from build123d import *

# Parameters (mm, degrees)
SKETCH_1_W          = 32
SKETCH_1_H          = 34
SKETCH_1_R          = 3.388194149
SKETCH_1_R_2        = 1.2
SKETCH_1_R_3        = 5.5
EXTRUDE_1_DEPTH     = 13.5
EXTRUDE_START       = 3
SKETCH_1_26_R       = 1.2
EXTRUDE_3_DEPTH     = 10.5
EXTRUDE_START_2     = -3
SKETCH_1_25_W       = 32
SKETCH_1_25_H       = 34
SKETCH_1_25_R       = 3.388194149
SKETCH_1_25_R_2     = 1.2
EXTRUDE_2_DEPTH     = 3
SKETCH_2_W          = 4
SKETCH_2_H          = 7
SKETCH_2_W_2        = 5
SKETCH_2_H_2        = 2
EXTRUDE_4_DEPTH     = 4
SKETCH_2_3_R        = 1.5
CUT_EXTRUDE_1_DEPTH = 35.091787867
CUT_EXTRUDE_START   = -16.5
SKETCH_2_4_R        = 2.25
CUT_EXTRUDE_2_DEPTH = 14.5
SKETCH_3_R          = 0.75
CUT_EXTRUDE_3_DEPTH = 4
SKETCH_1_27_R       = 3.388194149
EXTRUDE_5_DEPTH     = 16.5


with BuildPart() as part:
    # 草图1 → 凸台-拉伸1 (new body)
    with BuildSketch(Plane(origin=(0, 0, 0), x_dir=(1, 0, 0), z_dir=(0, 1, 0))):
        with Locations((3, 6)):
            Rectangle(SKETCH_1_W, SKETCH_1_H)
        with Locations(Location((11.473501894, 0, 0), (0, 0, 270))):
            Circle(SKETCH_1_R, mode=Mode.SUBTRACT)
        with Locations(Location((-3.489130435, 11.48154906, 0), (0, 0, 270))):
            Circle(SKETCH_1_R_2, mode=Mode.SUBTRACT)
        with Locations(Location((0, 0, 0), (0, 0, 270))):
            Circle(SKETCH_1_R_3, mode=Mode.SUBTRACT)
    extrude(amount=EXTRUDE_1_DEPTH)

    # 草图1<26> → 凸台-拉伸3 (add)
    with BuildSketch(Plane(origin=(0, 0, 0), x_dir=(1, 0, 0), z_dir=(0, 1, 0)).offset(EXTRUDE_START)):
        with Locations(Location((-3.489130435, 11.48154906, 0), (0, 0, 270))):
            Circle(SKETCH_1_26_R)
    extrude(amount=EXTRUDE_3_DEPTH)

    # 草图1<25> → 凸台-拉伸2 (add)
    with BuildSketch(Plane(origin=(0, 0, 0), x_dir=(1, 0, 0), z_dir=(0, 1, 0)).offset(EXTRUDE_START_2)):
        with Locations((3, 6)):
            Rectangle(SKETCH_1_25_W, SKETCH_1_25_H)
        with Locations(Location((11.473501894, 0, 0), (0, 0, 270))):
            Circle(SKETCH_1_25_R, mode=Mode.SUBTRACT)
        with BuildLine():
            ThreePointArc((5.276856444, 1.550737267), (6.181423335, 0.479588939), (5.452898061, -0.718263692))
            ThreePointArc((5.452898061, -0.718263692), (-1.935120147, -5.148330799), (-4.575965094, 3.051318314))
            ThreePointArc((-4.575965094, 3.051318314), (-5.960597826, 19.614312977), (2.104497703, 5.081445603))
            ThreePointArc((2.104497703, 5.081445603), (4.091157856, 3.67592538), (5.276856444, 1.550737267))
        make_face(mode=Mode.SUBTRACT)
        with Locations(Location((8.010869565, 11.48154906, 0), (0, 0, 270))):
            Circle(SKETCH_1_25_R_2, mode=Mode.SUBTRACT)
    extrude(amount=EXTRUDE_2_DEPTH)

    # 草图2 → 凸台-拉伸4 (add)
    with BuildSketch(Plane(origin=(0, 13.5, 0), x_dir=(1, 0, 0), z_dir=(0, 1, 0))):
        with Locations((-15, 9.3)):
            Rectangle(SKETCH_2_W, SKETCH_2_H)
        with Locations((0.1, -12)):
            Rectangle(SKETCH_2_W_2, SKETCH_2_H_2)
    extrude(amount=-EXTRUDE_4_DEPTH)

    # 草图2<3> → 切除-拉伸1 (cut, through all)
    with BuildSketch(Plane(origin=(0, 13.5, 0), x_dir=(1, 0, 0), z_dir=(0, 1, 0))):
        with Locations(Location((-13.25, 9.25, 0), (0, 0, 270))):
            Circle(SKETCH_2_3_R)
        with Locations(Location((0, -9.25, 0), (0, 0, 270))):
            Circle(SKETCH_2_3_R)
        with Locations(Location((13.25, 9.25, 0), (0, 0, 270))):
            Circle(SKETCH_2_3_R)
    extrude(amount=-CUT_EXTRUDE_1_DEPTH, mode=Mode.SUBTRACT)

    # 草图2<4> → 切除-拉伸2 (cut)
    with BuildSketch(Plane(origin=(0, 13.5, 0), x_dir=(1, 0, 0), z_dir=(0, 1, 0)).offset(CUT_EXTRUDE_START)):
        with Locations(Location((-13.25, 9.25, 0), (0, 0, 83.620629792))):
            Circle(SKETCH_2_4_R)
        with Locations(Location((13.25, 9.25, 0), (0, 0, 270))):
            Circle(SKETCH_2_4_R)
        with Locations(Location((0, -9.25, 0), (0, 0, 308.942441269))):
            Circle(SKETCH_2_4_R)
    extrude(amount=CUT_EXTRUDE_2_DEPTH, mode=Mode.SUBTRACT)

    # 草图3 → 切除-拉伸3 (cut)
    with BuildSketch(Plane.XZ.offset(3)):
        with Locations(Location((-10, 8, 0), (0, 0, 270))):
            Circle(SKETCH_3_R)
        with Locations(Location((17, -21, 0), (0, 0, 270))):
            Circle(SKETCH_3_R)
        with Locations(Location((16, 8, 0), (0, 0, 270))):
            Circle(SKETCH_3_R)
    extrude(amount=-CUT_EXTRUDE_3_DEPTH, mode=Mode.SUBTRACT)

    # 草图1<27> → 凸台-拉伸5 (add, through all)
    with BuildSketch(Plane(origin=(0, 0, 0), x_dir=(1, 0, 0), z_dir=(0, 1, 0)).offset(EXTRUDE_START_2)):
        with Locations((11.473501894, 0)):
            Circle(SKETCH_1_27_R)
    extrude(amount=EXTRUDE_5_DEPTH)


solid = part.part
Could you check a few things on this model? Use its own coordinates, in mm. A direction names the side the tool comes from. Coordinates: 2 decimals unless noted, no trailing zeros. Order: outer loops, then holes, each group sorted by start corner. A loop starts at its lowest first (then second) coordinate and runs counter-clockwise, first axis right, second up.
Q1. Which directions (+Z, -Z, +X, -X, +Y, -Y) give clear straight access to the entire face, cutting with the end or side of a thin tool? Please do faces 1 (the cylindrical face through (-13.18, 12.51, -10.75)), 2 (the flat face through (-2.4, 12, 12)), 3 (the cylindrical face through (9.2, -1.52, -11.64)), 4 (the flat face through (2.6, 12, 12)), 5 (the flat face through (-15, 12, -12.8)).
Q2. Thinking about a two-plate mould opening in Z: for faces 6 (the flat face through (0, 12, 13)), 7 (the flat face through (5, 13.5, -5)), 8 (the cylindrical face through (6.18, -1.52, -0.5)), which applies, released by +Z, released by -Z, zero draft, split by the parting line, or undercut?
Q3. Please list where these lines run through material, in increasing order: L1, parallel to Z at x = 0, y = 10; L2, parallel to X at y = 0.25, z = 8; L3, parallel to X at y = 2.5, z = 0.
Q4. Suppose I cut it at B-B on y = 5.75. Please give me the cut outline in (x, z).
Q5. Suppose I cut it at C-C on x = 13.25. Please give me the cut outline in (y, z).
Q6. Suppose I cut it at D-D on z = -9.25. Please give me the cut outline in (x, y).
Q7. Will these pins go through, and if not, where does the flat tip stop? pin 1 (2.5 mm diameter, centred on x = -3, z = -11.5, fed in from -Y); pin 2 (3 mm diameter, centred on x = 10, y = 10.5, fed in from +Z); pin 3 (2 mm diameter, centred on x = -15.5, z = -8, fed in from -Y).
Q8. Suppose I cut it at A-A on z = 9.25. Please give me the cut outline in (x, y), and give its area (3 significant figures).
Answer:
1. face 1: +Y, -Y
1. face 2: +Z, -X, +Y, -Y
1. face 3: -Y
1. face 4: +Z, +X, +Y, -Y
1. face 5: -Z, -X, +Y, -Y
2. face 6: released by +Z
2. face 7: zero draft
2. face 8: undercut
3. L1: z = -23 to -5.5, 5.5 to 7, 11.5 to 13
3. L2: x = -13 to -10.75, -9.25 to -1.87, 1.87 to 15.25, 16.75 to 19
3. L3: x = -13 to -5.5, 5.5 to 19
4. outline: (-13, -23) - (19, -23) - (19, 11) - (1.41, 11) arc R2.25 cw (long way) to (-1.41, 11) - (-13, 11) - (-13, -7.01) arc R2.25 cw to (-13, -11.49) - close; hole circle Ø11 at (0, 0); hole circle Ø4.5 at (13.25, -9.25)
5. outline: (-3, -23) - (13.5, -23) - (13.5, -10.75) - (11.5, -10.75) - (11.5, -11.5) - (-3, -11.5) - close; (-3, -7) - (11.5, -7) - (11.5, -7.75) - (13.5, -7.75) - (13.5, 11) - (-3, 11) - close
6. outline: (-17, 9.5) - (-15.5, 9.5) - (-15.5, 11.5) - (-14.75, 11.5) - (-14.75, 13.5) - (-17, 13.5) - close; (-11.75, 11.5) - (-11, 11.5) - (-11, 0) - (4.71, 0) - (4.71, -3) - (11, -3) - (11, 11.5) - (11.75, 11.5) - (11.75, 13.5) - (-11.75, 13.5) - close; (14.75, 11.5) - (15.5, 11.5) - (15.5, -3) - (19, -3) - (19, 13.5) - (14.75, 13.5) - close
7. pin 1: stops at y = 0
7. pin 2: stops at z = 11
7. pin 3: stops at y = 9.5
8. outline: (-13, -3) - (-2.25, -3) - (-2.25, 11.5) - (-1.5, 11.5) - (-1.5, 13.5) - (-13, 13.5) - close; (1.5, 11.5) - (2.25, 11.5) - (2.25, -3) - (19, -3) - (19, 13.5) - (1.5, 13.5) - close
8. area: 457 mm2
